from build123d import *

# Parameters (mm, degrees)
F1_DEPTH = 12.7


with BuildPart() as f1:
    # F0 (on Top) → F1 (new body)
    with BuildSketch(Plane.XY):
        Polygon((-418.2990551353, 237.649252063), (-419.9009448647, 237.649252063), (-419.9009448647, -346.550747937), (-354.444026947, -346.550747937), (-354.444026947, -301.0607462526), (-292.6674187183, -301.0607462526), (-292.6674187183, -346.550747937), (-76.3335824013, -346.550747937), (-76.3335824013, -114.4193708897), (76.3335824013, -114.4193708897), (76.3335824013, -346.550747937), (292.6674187183, -346.550747937), (292.6674187183, -301.0607462526), (354.444026947, -301.0607462526), (354.444026947, -346.550747937), (418.2990551353, -346.550747937), (418.2990551353, -270.350747937), (208.7490551353, -270.350747937), (208.7490551353, 161.449252063), (418.2990551353, 161.449252063), (418.2990551353, 237.649252063), (354.444026947, 237.649252063), (354.444026947, 192.1592503786), (292.6674187183, 192.1592503786), (292.6674187183, 237.649252063), (76.3335824013, 237.649252063), (76.3335824013, 5.5178750157), (-76.3335824013, 5.5178750157), (-76.3335824013, 237.649252063), (-292.6674187183, 237.649252063), (-292.6674187183, 192.1592503786), (-354.444026947, 192.1592503786), (-354.444026947, 237.649252063), align=None)
    extrude(amount=F1_DEPTH)


solid = f1.part
Work out the finished part from the listing and answer in its coordinate system (mm). Round coordinates to 2 decimals unless told otherwise and drop trailing zeros. Write each loop counter-clockwise with the first axis right and the second up, starting at its lowest first coordinate (ties: lowest second). Pieces come first, ordered by that corner, then holes. Notation, with made-up numbers: (45.5, 22) -> (84.5, 22) arc R21 ccw to (84.5, 31) -> close; hole circle Ø1 at (63, 43). An arc over 180 degrees is marked (long way). Answer as CSV lines item,"result". Start each with the question number.
(1) The part is cut by section A-A, the plane y = 67. Give the vertices of the cut face in (x, z), then the cut area to 4 significant figures.
(2) Find the intervals of material crossed by probe 1 along X at (y, z) = (-302, 8.5); probe 2 along Y at (x, z) = (336.5, 2); probe 3 along X at (y, z) = (56.5, 7), in increasing order.
(3) Each of these flat-tipped pins is pushed along its axis until it touches: pin 1 (4 mm diameter, centred on y = -187, z = 3.5, fed in from +X); pin 2 (1 mm diameter, centred on x = -17.5, z = 9.5, fed in from -Y); pin 3 (6.5 mm diameter, centred on x = 318, z = 6.5, fed in from -Y). Where does it stop, or does it pass through?
(4) The part is cut by section C-C, the plane x = -5.5. Give the vertices of the cut face in (y, z), then the cut area to 3 significant figures.
(5) The part is cut by section D-D, the plane y = -41. Give the vertices of the cut face in (x, z), then the cut area to 3 significant figures.
Output values:
1,outline,"(-419.9, 0) -> (-76.33, 0) -> (-76.33, 12.7) -> (-419.9, 12.7) -> close; (76.33, 0) -> (208.75, 0) -> (208.75, 12.7) -> (76.33, 12.7) -> close"
1,area,"6,045 mm²"
2,probe 1,"x = -419.9 to -354.44, -292.67 to -76.33, 76.33 to 292.67, 354.44 to 418.3"
2,probe 2,"y = -301.06 to -270.35, 161.45 to 192.16"
2,probe 3,"x = -419.9 to -76.33, 76.33 to 208.75"
3,pin 1,"stops at x = 208.75"
3,pin 2,"stops at y = -114.42"
3,pin 3,"stops at y = -301.06"
4,outline,"(-114.42, 0) -> (5.52, 0) -> (5.52, 12.7) -> (-114.42, 12.7) -> close"
4,area,"1,520 mm²"
5,outline,"(-419.9, 0) -> (208.75, 0) -> (208.75, 12.7) -> (-419.9, 12.7) -> close"
5,area,"7,980 mm²"
